CAD build for the part. Positions are in the model's coordinates, mm. A direction names the side the tool comes from. Give positions to 0.01 mm unless a question says otherwise; leave off trailing zeros. Write each loop counter-clockwise with the first axis right and the second up, starting at its lowest first coordinate (ties: lowest second). Pieces come first, ordered by that corner, then holes. Notation, with made-up numbers: (69, 51.5) - (116, 51.5) arc R22 ccw to (116, 69.5) - close; hole circle Ø6 at (56.25, 2.25). An arc over 180 degrees is marked (long way). Answer as a JSON object with one key per item and string values.
from build123d import *

# Parameters (mm, degrees)
F0_W     = 890
F0_H     = 724
F1_DEPTH = 20
F2_W     = 20
F2_H     = 724
F3_DEPTH = 48
F4_W     = 20
F4_H     = 724
F5_DEPTH = 48
F6_SIZE  = 4.9999


# Not quite as in the source:
# - a fillet or chamfer is up to 0.001 mm smaller than in the source, because OpenCascade refuses the exact size


with BuildPart() as f1:
    # F0 (on Front) → F1 (new body)
    with BuildSketch(Plane.XZ):
        with Locations((5.1721642405, -1.2866072357)):
            Rectangle(F0_W, F0_H)
    extrude(amount=F1_DEPTH)

    # F2 (on face) → F3 (join)
    with BuildSketch(Plane(origin=(-439.8278357595, 0, 0), x_dir=(0, -1, 0), z_dir=(-1, 0, 0))):
        Polygon((33, 365.7133927643), (-13, 365.7133927643), (-13, -363.2866072357), (0, -363.2866072357), (0, 360.7133927643), (20, 360.7133927643), (20, -363.2866072357), (33, -363.2866072357), align=None)
        with Locations((10, -1.2866072357)):
            Rectangle(F2_W, F2_H)
    extrude(amount=F3_DEPTH)

    # F4 (on face) → F5 (join)
    with BuildSketch(Plane.YZ.offset(450.1721642405)):
        with Locations((-10, -1.2866072357)):
            Rectangle(F4_W, F4_H)
        Polygon((13, 365.7133927643), (-33, 365.7133927643), (-33, -363.2866072357), (-20, -363.2866072357), (-20, 360.7133927643), (0, 360.7133927643), (0, -363.2866072357), (13, -363.2866072357), align=None)
    extrude(amount=F5_DEPTH)

    # F6 (size 5 in the source; OpenCascade refuses exactly that, so slightly less here)
    f6_edges = [f1.edges().sort_by_distance(p)[0] for p in [
        (-463.827836, -33, 365.713393),
        (-487.827836, -10, 365.713393),
        (-439.827836, -10, 365.713393),
        (-463.827836, 13, 365.713393),
        (5.172164, -20, 360.713393),
        (5.172164, 0, 360.713393),
        (474.172164, 13, 365.713393),
        (450.172164, -10, 365.713393),
        (474.172164, -33, 365.713393),
        (498.172164, -10, 365.713393),
        (-487.827836, 13, 1.213393),
        (-439.827836, 13, 1.213393),
        (-487.827836, -33, 1.213393),
        (-439.827836, -33, 1.213393),
        (450.172164, -33, 1.213393),
        (474.172164, -33, -363.286607),
        (498.172164, -33, 1.213393),
        (450.172164, 13, 1.213393),
        (498.172164, 13, 1.213393),
    ]]
    chamfer(f6_edges, length=F6_SIZE)


solid = f1.part
Item 1: Mould opens along X. For faces 1 (the flat face through (-439.828, -22, 4)), 2 (the flat face through (-2, -10, -363.287)), 3 (the flat face through (498.172, -10, 4)), 4 (the flat face through (-1, -20, 1)) say: +X half, -X half, draft (parallel to the pull), parting line (faces both ways), or undercut.
Entries:
{"face 1": "undercut", "face 2": "draft", "face 3": "+X half", "face 4": "undercut"}
Item 2: Cut at A-A (z = -244.5). Give the cut face in (x, y).
Entries:
{"outline": "(-487.83, -28) - (-482.83, -33) - (-444.83, -33) - (-439.83, -28) - (-439.83, -20) - (450.17, -20) - (450.17, -28) - (455.17, -33) - (493.17, -33) - (498.17, -28) - (498.17, 8) - (493.17, 13) - (455.17, 13) - (450.17, 8) - (450.17, 0) - (-439.83, 0) - (-439.83, 8) - (-444.83, 13) - (-482.83, 13) - (-487.83, 8) - close"}
Item 3: Cut at B-B (x = -305.5). Give the cut face in (y, z).
Entries:
{"outline": "(-20, -363.29) - (0, -363.29) - (0, 355.71) - (-5, 360.71) - (-15, 360.71) - (-20, 355.71) - close"}
Item 4: Flat gauge pins, fed straight in: P1, Ø8, axis at x = -134.5, y = -8, coming from the +Z side; P2, Ø5, axis at x = 117, z = -45, coming from the -Y side; P3, Ø8, axis at x = 10.5, z = -197.5, coming from the +Y side. Where does each tip first touch, or does it go through?
Entries:
{"P1": "z = 360.71", "P2": "y = -20", "P3": "y = 0"}
Item 5: Probe line 1 (X direction, y = 8, z = -313.5); line 2 (Y direction, x = 390, z = -280); line 3 (X direction, y = -30.5, z = -50.5). List the from-to ranges inside material, lowest first. Write a range as from..to.
Entries:
{"line 1": "-487.83..-439.83, 450.17..498.17", "line 2": "-20..0", "line 3": "-485.33..-442.33, 452.67..495.67"}
Item 6: Which spindle directions (+Z, -Z, +X, -X, +Y, -Y) get a long thin tool onto all of the face, cutting with end or side? Do faces 5 (the flat face through (-1, 0, 1)), 6 (the flat face through (-487.828, -10, 4)). Say none if no direction does.
Entries:
{"face 5": "+Z, -Z, +Y", "face 6": "+Z, -Z, -X, +Y, -Y"}
